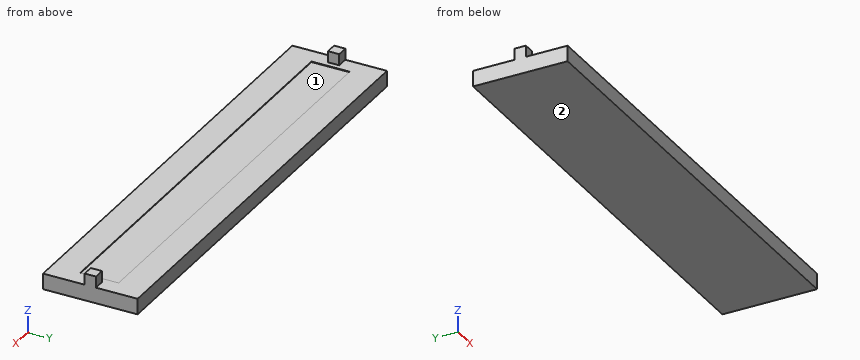
```python
from build123d import *

# Parameters (mm, degrees)
F0_W     = 205
F0_H     = 42
F1_DEPTH = 7
F2_W     = 5
F2_H     = 5
F3_DEPTH = 5
F2_W_2   = 190
F2_H_2   = 17
F4_DEPTH = 0.25


with BuildPart() as f1:
    # F0 (on Top) → F1 (new body)
    with BuildSketch(Plane.XY):
        with Locations((0, -26.665802)):
            Rectangle(F0_W, F0_H)
    extrude(amount=F1_DEPTH)

    # F2 (on face) → F3 (join)
    with BuildSketch(Plane.XY.offset(7)):
        with Locations((-100, -26.665802)):
            Rectangle(F2_W, F2_H)
        with Locations((100, -26.665802)):
            Rectangle(F2_W, F2_H)
    extrude(amount=F3_DEPTH)

    # F2 (on face) → F4 (cut)
    with BuildSketch(Plane.XY.offset(7)):
        with Locations((0, -26.665802)):
            Rectangle(F2_W_2, F2_H_2)
    extrude(amount=-F4_DEPTH, mode=Mode.SUBTRACT)


solid = f1.part
```
The model under review builds one solid part; all positions refer to its coordinate system, in mm. Face numbers are marked on the shaded views. Coordinates: 2 decimals unless noted, no trailing zeros. Order: outer loops, then holes, each group sorted by start corner. A loop starts at its lowest first (then second) coordinate and runs counter-clockwise, first axis right, second up. Notation, with made-up numbers: M 32,36 L 38,36 A19 cw 38,41 Z; hole C 34,12 d10. An arc over 180 degrees is marked long. One line per question, with ' | ' between items.
(1) Add section B-B, the plane x = 70.5. Write out the cut boundary in (y, z).
Geometry results:
outline: M -47.67,0 L -5.67,0 L -5.67,7 L -18.17,7 L -18.17,6.75 L -35.17,6.75 L -35.17,7 L -47.67,7 Z
(2) Add section A-A, the plane z = 9. Write out the cut boundary in (x, y).
Geometry results:
outline: M -102.5,-29.17 L -97.5,-29.17 L -97.5,-24.17 L -102.5,-24.17 Z; M 97.5,-29.17 L 102.5,-29.17 L 102.5,-24.17 L 97.5,-24.17 Z
(3) Insertion check: pin 1 (13.5 mm diameter, centred on x = -15.5, y = -27.5, fed in from +Z); pin 2 (4 mm diameter, centred on x = -99, z = 10.5, fed in from +Y); pin 3 (2.5 mm diameter, centred on x = -100.5, z = 10.5, fed in from -Y). Each pin has a flat end and moves straight along its axis. Give the tip position at first contact, or say it passes through.
Geometry results:
pin 1: stops at z = 6.75 | pin 2: stops at y = -24.17 | pin 3: stops at y = -29.17
(4) For probe 1 along Z at (x, y) = (-39.5, -45); probe 2 along Z at (x, y) = (-32.5, -30.5), list the stretches that pass through material, from the lowest coordinate up. Write a range as from..to.
Geometry results:
probe 1: z = 0..7 | probe 2: z = 0..6.75
(5) Add section C-C, the plane y = -37.5. Write out the cut boundary in (x, z).
Geometry results:
outline: M -102.5,0 L 102.5,0 L 102.5,7 L -102.5,7 Z
(6) The part is to be moulded in two halves that separate along Y. For the marked faces 1 and 2, say which applies: +Y half, -Y half, draft (parallel to the pull), parting line (faces both ways), or undercut.
Geometry results:
face 1: undercut | face 2: draft
